```python
from build123d import *

# Parameters (mm, degrees)
BOSS_EXTRUDE2_DEPTH     = 3
CUT_EXTRUDE3_DEPTH      = 108.193349502
CUT_EXTRUDE3_DEPTH_BACK = 108.193349502
SKETCH3_R               = 1.6
CUT_EXTRUDE4_DEPTH      = 108.193349502
CUT_EXTRUDE4_DEPTH_BACK = 108.193349502
SKETCH4_R               = 1.6


with BuildPart() as part:
    # Sketch1 → Boss-Extrude2 (new body)
    with BuildSketch(Plane(origin=(0, 0, 0), x_dir=(1, 0, 0), z_dir=(0, 1, 0))):
        Polygon((0, -75.76745402), (53.575680531, -53.575680531), (75.76745402, 0), (53.575680531, 53.575680531), (0, 75.76745402), (-53.575680531, 53.575680531), (-75.76745402, 0), (-53.575680531, -53.575680531), align=None)
    extrude(amount=BOSS_EXTRUDE2_DEPTH)

    # Sketch3 → Cut-Extrude3 (cut, two sides: drawn at the far end of the back side and taken through both)
    with BuildSketch(Plane(origin=(0, 3, 0), x_dir=(1, 0, 0), z_dir=(0, 1, 0)).offset(-CUT_EXTRUDE3_DEPTH_BACK)):
        with Locations(Location((-70.710678119, 0, 0), (0, 0, 270))):
            Circle(SKETCH3_R)
        with Locations(Location((0, 70.710678119, 0), (0, 0, 270))):
            Circle(SKETCH3_R)
        with Locations(Location((70.710678119, 0, 0), (0, 0, 270))):
            Circle(SKETCH3_R)
        with Locations(Location((0, -70.710678119, 0), (0, 0, 270))):
            Circle(SKETCH3_R)
    extrude(amount=CUT_EXTRUDE3_DEPTH + CUT_EXTRUDE3_DEPTH_BACK, mode=Mode.SUBTRACT)

    # Sketch4 → Cut-Extrude4 (cut, two sides: drawn at the far end of the back side and taken through both)
    with BuildSketch(Plane(origin=(0, 3, 0), x_dir=(1, 0, 0), z_dir=(0, 1, 0)).offset(-CUT_EXTRUDE4_DEPTH_BACK)):
        with Locations(Location((-19.891628757, -41, 0), (0, 0, 270))):
            Circle(SKETCH4_R)
        with Locations(Location((20.108371243, -41, 0), (0, 0, 270))):
            Circle(SKETCH4_R)
        with Locations(Location((-28, 29, 0), (0, 0, 270))):
            Circle(SKETCH4_R)
        with Locations(Location((28, 29, 0), (0, 0, 270))):
            Circle(SKETCH4_R)
    extrude(amount=CUT_EXTRUDE4_DEPTH + CUT_EXTRUDE4_DEPTH_BACK, mode=Mode.SUBTRACT)


solid = part.part
```
CAD build for the part. Positions are in the model's coordinates, mm. Round coordinates to 2 decimals unless told otherwise and drop trailing zeros. Order: outer loops, then holes, each group sorted by start corner. A loop starts at its lowest first (then second) coordinate and runs counter-clockwise, first axis right, second up. Notation, with made-up numbers: (-11.5, 0.25) - (28.5, 0.25) arc R15 cw to (28.5, 18.25) - close; hole circle Ø10 at (-31.75, 76). An arc over 180 degrees is marked (long way). Answer as CSV lines item,"result". Start each with the question number.
1. Saw through at B-B, the plane x = 32. Write the cut outline in (y, z).
2. Saw through at C-C, the plane z = -58. Write the cut outline in (x, y), and give its area (3 significant figures).
3. Drill centre lines: L1, parallel to X at y = 1.8, z = 0; L2, parallel to X at y = 1.3, z = -29. Where is each one in solid material? Low to high. Write a range as [from, to].
4. Saw through at A-A, the plane y = 2.45. Count the separate pieces of the cut face and the enclosed holes in it, and give its area (3 significant figures).
Model answer:
1,outline,"(0, -62.51) - (3, -62.51) - (3, 62.51) - (0, 62.51) - close"
2,outline,"(-42.89, 0) - (42.89, 0) - (42.89, 3) - (-42.89, 3) - close"
2,area,"257 mm²"
3,L1,"x = [-75.77, -72.31], [-69.11, 69.11], [72.31, 75.77]"
3,L2,"x = [-63.76, -29.6], [-26.4, 26.4], [29.6, 63.76]"
4,separate pieces,"1"
4,enclosed holes,"8"
4,area,"16,200 mm²"
